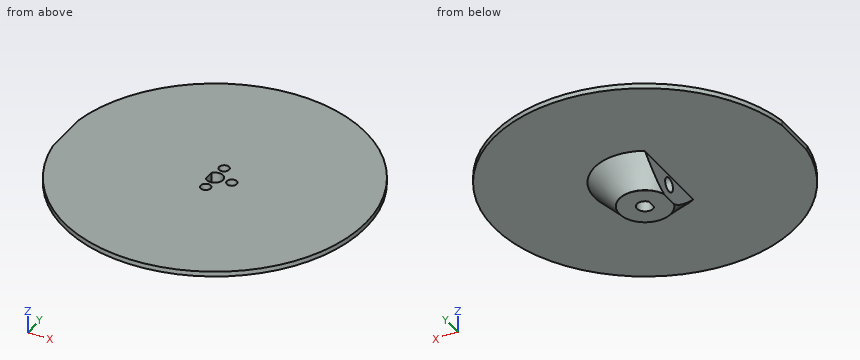
Autodesk Inventor part; units mm, degrees
ref_plane "YZ Plane" through (0, 0, 0) normal (1, 0, 0) x (0, 1, 0)
ref_plane "XZ Plane" through (0, 0, 0) normal (0, 1, 0) x (-1, 0, 0)
ref_plane "XY Plane" through (0, 0, 0) normal (0, 0, 1) x (1, 0, 0)
sketch "Sketch1" plane through (0, 0, 0) normal (0, 0, 1) x (1, 0, 0)
  arc A0 (-2.55, -2.0149) -> (-2.55, 2.0149) centre (0, 0) ccw
  line L0 (-2.55, 2.0149) -> (-2.55, -2.0149)
  arc A1 (-9.55, -3.7229) -> (-9.55, 3.7229) centre (0, 0) ccw
  line L1 (-9.55, -3.7229) -> (-9.55, 3.7229)
  point P0 (0, 0)
  dimension "d4" = 7
extrude "Extrusion1" add sketch "Sketch1" along normal blind 12
sketch "Sketch2" plane through (-9.55, -3.7229, 0) normal (-1, 0, 0) x (0, 0, 1)
  line L0 (0, 7.4458) -> (0, 0)
  line L1 (0, 0) -> (12, 0)
  line L2 (12, 7.4458) -> (12, 0)
  line L3 (0, 7.4458) -> (12, 7.4458)
  circle A0 centre (6, 3.7229) radius 3.25
  circle A1 centre (6, 3.7229) radius 2.85
  point P0 (0, 3.7229)
  dimension "d15" = 5.7
extrude "Extrusion2" cut sketch "Sketch2" against normal blind 10.4125 contours A1
sketch "Sketch3" plane through (0, 0, 12) normal (0, 0, 1) x (1, 0, 0)
  arc A0 (-2.55, -2.0149) -> (-2.55, 2.0149) centre (0, 0) ccw
  line L0 (-2.55, 2.0149) -> (-2.55, -2.0149)
  line L1 (-9.55, 3.7229) -> (-9.55, -3.7229)
  arc A1 (-9.55, -3.7229) -> (-9.55, 3.7229) centre (0, 0) ccw
  line L2 (-2.55, -2.0149) -> (-2.55, 2.0149)
  arc A2 (-2.55, -2.0149) -> (-2.55, 2.0149) centre (0, 0) ccw
  line L3 (0, 10.25) -> (0, 3.25)
  circle A3 centre (0, 6.75) radius 2
  circle A4 centre (6.75, 0) radius 2
  circle A5 centre (0, -6.75) radius 2
  point P0 (0, 0)
  dimension "d7" = 4
  dimension "d10" = 180
extrude "Extrusion3" cut sketch "Sketch3" against normal blind 5.7 contours A3 L3 | L3 A3 | A4 | A5
sketch "Sketch4" plane through (0, 0, 12) normal (0, 0, 1) x (1, 0, 0)
  circle A0 centre (0, -6.75) radius 2
  circle A1 centre (6.75, 0) radius 2
  circle A2 centre (0, 6.75) radius 2
  line L0 (-9.55, 3.7229) -> (-9.55, -3.7229)
  arc A3 (-9.55, -3.7229) -> (-9.55, 3.7229) centre (0, 0) ccw
  line L1 (-2.55, -2.0149) -> (-2.55, 2.0149)
  arc A4 (-2.55, -2.0149) -> (-2.55, 2.0149) centre (0, 0) ccw
  line L2 (-59.55, -9.1575) -> (-59.55, 9.1575)
  arc A5 (-59.55, -9.1575) -> (-59.55, 9.1575) centre (0, 0) ccw
  point P0 (0, 0)
  dimension "d16" = 50
extrude "Extrusion4" add sketch "Sketch4" against normal blind 2 contours L2 A5
chamfer "Chamfer1" distance 9.9375 angle 45 1 edges at (10.25, 0, 10)
properties part number "Pladeholder"
Here's how the part is built. I have some questions about the finished solid (model axes, mm). Round coordinates to 2 decimals unless told otherwise and drop trailing zeros. Order: outer loops, then holes, each group sorted by start corner. A loop starts at its lowest first (then second) coordinate and runs counter-clockwise, first axis right, second up. Notation, with made-up numbers: (61.25, -6.5) -> (117.25, -6.5) arc R30 cw to (117.25, 29.5) -> close; hole circle Ø7 at (-19, 8.25). An arc over 180 degrees is marked (long way). Return JSON: item names as keys, results as strings.
Q1. If we section it at B-B on y = 47: List the corners of the cut face in (x, z) for me.
Filled sheet:
{"outline": "(-37.7, 10) -> (37.7, 10) -> (37.7, 12) -> (-37.7, 12) -> close"}
Q2. If we section it at A-A on x = 0: List the corners of the cut face in (y, z) for me, plus the area to 3 significant figures.
Filled sheet:
{"outline": "(-60.25, 10) -> (-20.19, 10) -> (-10.25, 0.06) -> (-10.25, 0) -> (-3.25, 0) -> (-3.25, 12) -> (-4.75, 12) -> (-4.75, 6.3) -> (-8.75, 6.3) -> (-8.75, 12) -> (-60.25, 12) -> close; (3.25, 0) -> (10.25, 0) -> (10.25, 0.06) -> (20.19, 10) -> (60.25, 10) -> (60.25, 12) -> (8.75, 12) -> (8.75, 6.3) -> (4.75, 6.3) -> (4.75, 12) -> (3.25, 12) -> close", "area": "421 mm^2"}
Q3. For pin 1 Ø4 at (x, y) = (-25, -0.5) entering from -Z; pin 2 Ø3 at (x, y) = (0, -7) entering from +Z; pin 3 Ø1.2 at (y, z) = (0.5, 2) entering from +X, each with a flat end and sliding along its axis, tell me the tip position at first contact or that it passes through.
Filled sheet:
{"pin 1": "stops at z = 10", "pin 2": "stops at z = 6.3", "pin 3": "stops at x = 12.78"}
Q4. I need wall thicknesses on line 1 along Y through (x, z) = (0, 10.2); line 2 along Y through (x, z) = (0, 9.9); line 3 along Z through (x, y) = (-7, 0). Which ranges of each line are inside material? Lowest first, please. Write a range as from..to.
Filled sheet:
{"line 1": "y = -60.25..-8.75, -4.75..-3.25, 3.25..4.75, 8.75..60.25", "line 2": "y = -20.09..-8.75, -4.75..-3.25, 3.25..4.75, 8.75..20.09", "line 3": "z = 0..3.15, 8.85..12"}
Q5. If we section it at C-C on x = -27: List the corners of the cut face in (y, z) for me.
Filled sheet:
{"outline": "(-53.86, 10) -> (53.86, 10) -> (53.86, 12) -> (-53.86, 12) -> close"}
